Read the model definition and answer for the solid it produces. Units are mm, in the model's axes. A direction names the side the tool comes from. Coordinates: 2 decimals unless noted, no trailing zeros. Order: outer loops, then holes, each group sorted by start corner. A loop starts at its lowest first (then second) coordinate and runs counter-clockwise, first axis right, second up. Notation, with made-up numbers: (-22.5, -31.5) - (-10.5, -31.5) arc R21 ccw to (-10.5, 3.5) - close; hole circle Ø9 at (-6, 10.25). An arc over 180 degrees is marked (long way). Answer as a JSON object with one key per item and string values. Group by question number.
from build123d import *

# Parameters (mm, degrees)
FILLET1_R = 0.5
FILLET2_R = 0.5
FILLET3_R = 0.5


with BuildPart() as part:
    # Sketch1 → Revolve1 (revolve)
    with BuildSketch(Plane(origin=(0, 0, 0), x_dir=(1, 0, 0), z_dir=(0, 1, 0)), mode=Mode.PRIVATE) as revolve1_sk:
        Polygon((0, 0), (27.1, 0), (27.1, 3.6), (24.5, 3.6), (24.5, 2.75), (0, 2.75), align=None)
    revolve(revolve1_sk.sketch.rotate(Axis((0, 0, 0), (1, 0, 0)), 180), axis=Axis((0, 0, 0), (1, 0, 0)))

    # Fillet1
    fillet1_edges = [part.edges().sort_by_distance(p)[0] for p in [
        (27.1, 0, -3.6),
    ]]
    fillet(fillet1_edges, radius=FILLET1_R)

    # Fillet2
    fillet2_edges = [part.edges().sort_by_distance(p)[0] for p in [
        (0, 0, -2.75),
    ]]
    fillet(fillet2_edges, radius=FILLET2_R)

    # Fillet3
    fillet3_edges = [part.edges().sort_by_distance(p)[0] for p in [
        (24.5, 0, -3.6),
    ]]
    fillet(fillet3_edges, radius=FILLET3_R)


solid = part.part
1. Straight lines are drawn through the part: L1, parallel to Y at x = 18.25, z = 0; L2, parallel to X at y = 1.25, z = -2.75; L3, parallel to Y at x = 22.5, z = -1. For each, find the intervals that lie inside material, in ascending order.
2. A cutting plane is placed at C-C on x = 17.5. Write down the section's boundary in (y, z).
3. A cutting plane is placed at A-A on z = 0. Write down the section's boundary in (x, y), and give its area (3 significant figures).
4. For faces 1 (the cylindrical face through (12.332, 2.685, -0.596)), 2 (the flat face through (0, 0, 0)), determine the directions among +Z, -Z, +X, -X, +Y, -Y from which every point of the face is accessible in a straight line to the end or side of a thin tool.
5. Given pin 1 (3 mm diameter, centred on x = 4.5, z = 2.5, fed in from -Y); pin 2 (4 mm diameter, centred on x = 8, z = 2, fed in from +Y); pin 3 (1 mm diameter, centred on x = 10.5, y = -1.5, fed in from -Z), each flat-ended and moving along its own axis, determine where each tip first touches the part or whether it passes through.
Derived:
{
 "1": {"L1": "y = -2.75 to 2.75", "L2": "x = 24.5 to 27.1", "L3": "y = -2.56 to 2.56"},
 "2": {"outline": "circle Ø5.5 at (0, 0)"},
 "3": {"outline": "(0, -2.25) arc R0.5 ccw to (0.5, -2.75) - (24.5, -2.75) - (24.5, -3.1) arc R0.5 ccw to (25, -3.6) - (26.6, -3.6) arc R0.5 ccw to (27.1, -3.1) - (27.1, 3.1) arc R0.5 ccw to (26.6, 3.6) - (25, 3.6) arc R0.5 ccw to (24.5, 3.1) - (24.5, 2.75) - (0.5, 2.75) arc R0.5 ccw to (0, 2.25) - close", "area": "153 mm2"},
 "4": {"face 1": "-X", "face 2": "+Z, -Z, -X, +Y, -Y"},
 "5": {"pin 1": "stops at y = -2.56", "pin 2": "stops at y = 2.75", "pin 3": "stops at z = -2.56"}
}
